```python
from build123d import *

# Parameters (mm, degrees)
F0_R     = 22.389121
F1_DEPTH = 20.32
F2_R     = 14.925471
F3_DEPTH = 20.321
F4_W     = 32.802565
F4_H     = 20.843296
F5_DEPTH = 5.588
F6_W     = 4.409732
F6_H     = 14.755644
F7_DEPTH = 16.764
F9_DEPTH = 50.486326


with BuildPart() as f1:
    # F0 (on Top) → F1 (new body)
    with BuildSketch(Plane.XY):
        with Locations((36.225565, 28.096205)):
            Circle(F0_R)
    extrude(amount=F1_DEPTH)

    # F2 (on Top) → F3 (cut, through all)
    with BuildSketch(Plane.XY):
        with Locations((35.655081, 28.096205)):
            Circle(F2_R)
    extrude(amount=F3_DEPTH, mode=Mode.SUBTRACT)

    # F4 (on Top) → F5 (join)
    with BuildSketch(Plane.XY):
        with Locations((-0.175342, 26.411418)):
            Rectangle(F4_W, F4_H)
    extrude(amount=F5_DEPTH)

    # F6 (on Right) → F7 (join)
    with BuildSketch(Plane.YZ):
        with Locations((28.172397, 12.87685)):
            Rectangle(F6_W, F6_H)
    extrude(amount=F7_DEPTH)

    # F8 (on Front) → F9 (cut, through all)
    with BuildSketch(Plane.XZ):
        Polygon((0, 5.684014), (13.850843, 20.343132), (0, 20.852523), align=None)
    extrude(amount=-F9_DEPTH, mode=Mode.SUBTRACT)


solid = f1.part
```
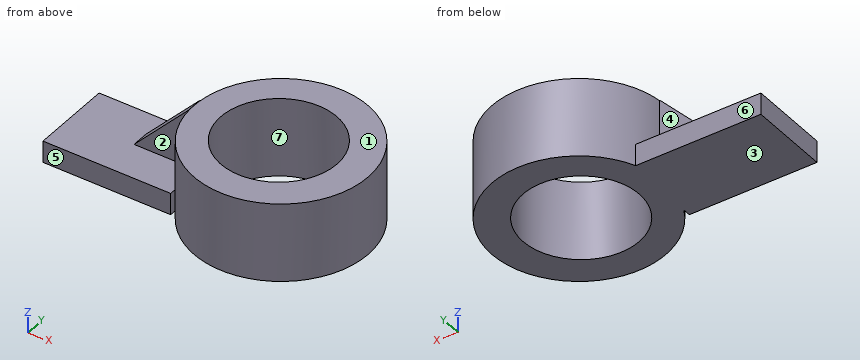
Geometry check sheet. Reference: the model listing, model coordinates, mm. Face numbers are marked on the shaded views. A direction names the side the tool comes from. Round coordinates to 2 decimals unless told otherwise and drop trailing zeros. Order: outer loops, then holes, each group sorted by start corner. A loop starts at its lowest first (then second) coordinate and runs counter-clockwise, first axis right, second up. Notation, with made-up numbers: (39.5, 24.5) -> (70.5, 24.5) arc R24 cw to (70.5, 36.5) -> close; hole circle Ø4 at (64.5, 13.5). An arc over 180 degrees is marked (long way). Return JSON: item names as keys, results as strings. Group by question number.
Q1. Section check C-C, the plane z = 11.5. Record the boundary of the cut face in (x, y).
Q2. Section check A-A, the plane y = 39.5. Record the boundary of the cut face in (x, z), plus the area to 3 significant figures.
Q3. Release check for a two-part mould opening along X. For the marked faces 6 and 7 record: released by +X, released by -X, zero draft, split by the parting line, or undercut.
Q4. Section check D-D, the plane x = 8. Record the boundary of the cut face in (y, z), plus the area to 3 significant figures.
Q5. Material ranges on probe 1 along Y at (x, z) = (35.5, 2.5); probe 2 along Z at (x, y) = (3, 35); probe 3 along Y at (x, z) = (9, 15), recorded low to high. Write a range as from..to.
Q6. Gauge pin test, flat ends, axial feed: pin 1 (8 mm diameter, centred on x = 25, z = 16.5, fed in from +Y); pin 2 (6 mm diameter, centred on y = 13, z = 9, fed in from +X); pin 3 (1 mm diameter, centred on y = 38.5, z = 9, fed in from -X). Record the tip position at first contact, or that the pin passes through.
Q7. Section check B-B, the plane x = 22. Record the boundary of the cut face in (y, z).
Q8. Tool access check on the marked faces 1, 2, 3, 4 and 5. Record the directions out of +Z, -Z, +X, -X, +Y, -Y that give a thin tool (end or side, any length) a straight path to the whole face; none if there is none.
Numbers:
{
 "1": {"outline": "(5.5, 25.97) -> (13.94, 25.97) arc R22.39 ccw (long way) to (13.95, 30.38) -> (5.5, 30.38) -> close; hole circle Ø29.85 at (35.66, 28.1)"},
 "2": {"outline": "(16.96, 0) -> (26.03, 0) -> (26.03, 20.32) -> (16.96, 20.32) -> close; (45.28, 0) -> (55.49, 0) -> (55.49, 20.32) -> (45.28, 20.32) -> close", "area": "392 mm^2"},
 "3": {"face 6": "zero draft", "face 7": "undercut"},
 "4": {"outline": "(15.99, 0) -> (36.83, 0) -> (36.83, 5.59) -> (30.38, 5.59) -> (30.38, 14.15) -> (25.97, 14.15) -> (25.97, 5.59) -> (15.99, 5.59) -> close", "area": "154 mm^2"},
 "5": {"probe 1": "5.72..13.17, 43.02..50.47", "probe 2": "0..5.59", "probe 3": "25.97..30.38"},
 "6": {"pin 1": "y = 49.29", "pin 2": "x = 55.07", "pin 3": "x = 16.15"},
 "7": {"outline": "(10.81, 0) -> (22.07, 0) -> (22.07, 20.32) -> (10.81, 20.32) -> close; (34.12, 0) -> (45.39, 0) -> (45.39, 20.32) -> (34.12, 20.32) -> close"},
 "8": {"face 1": "+Z, +X, -X, +Y, -Y", "face 2": "+Z, -X, -Y", "face 3": "-Z, +X, -X, +Y, -Y", "face 4": "+Z, -X, +Y", "face 5": "+Z, -Z, -X, -Y"}
}
